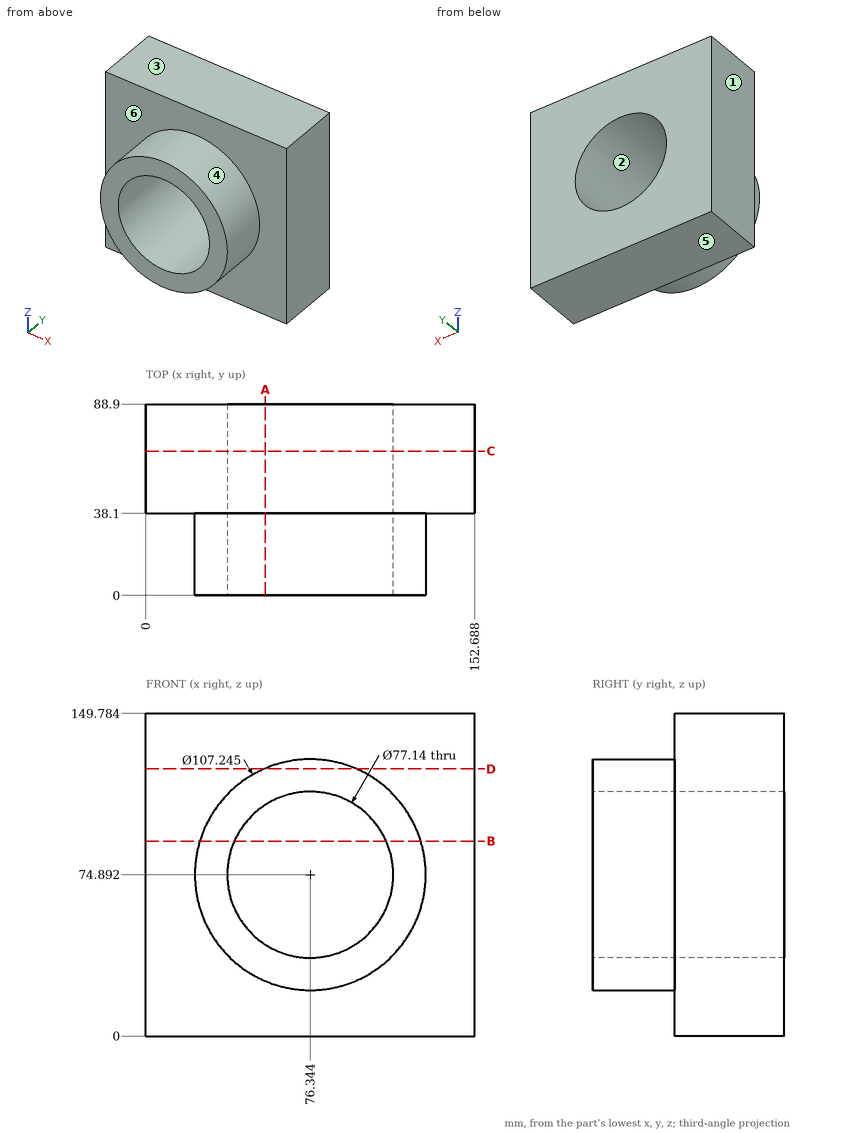
Can you work these out from the drawing? Everything is in mm from the part's minimum corner. A direction names the side the tool comes from. Coordinates: 2 decimals unless noted, no trailing zeros. Write each loop counter-clockwise with the first axis right and the second up, starting at its lowest first coordinate (ties: lowest second). Pieces come first, ordered by that corner, then holes. Notation, with made-up numbers: (39, 48) -> (55, 48) arc R15 cw to (55, 71) -> close; hole circle Ø10 at (82.25, 48.25). An arc over 180 degrees is marked (long way). Write each question's results on one line, items separated by ' | '. Start each with the question number.
Q1. Imagine slicing it at B-B (z = 90.5). Write out the boundary of the cut face in (x, y) (1 decimal).
Q2. If I drill on probe 1 along Z at (x, y) = (75.5, 28); probe 2 along Y at (x, z) = (75.5, 20); probe 3 along X at (y, z) = (56.5, 61) (1 decimal), over which ranges is the centre line in solid material (lowest first)?
Q3. Imagine slicing it at C-C (y = 67). Write out the boundary of the cut face in (x, z) (1 decimal), then the cut area to 3 significant figures.
Q4. Imagine slicing it at D-D (z = 124). Write out the boundary of the cut face in (x, y).
Q5. Imagine slicing it at A-A (x = 55.5). Write out the boundary of the cut face in (y, z) (1 decimal).
Q6. I'm going to push flat-ended pins straight in: pin 1 (8 mm diameter, centred on y = 13, z = 126.5, fed in from +X); pin 2 (5 mm diameter, centred on y = 12, z = 75, fed in from +X). Where does each tip first touch, or does it pass through?
Q7. On a 3-axis mill with a long thin cutter (end or side, diameter ignored), from which of +Z, -Z, +X, -X, +Y, -Y can I reach the whole of each face in a straight line? I mean the marked faces 5 and 6. Say none if no direction works.
Q8. We'd pull the mould along X, two halves only. Please class the marked faces 1, 2, 3 and 4: +X half, -X half, draft (parallel to the pull), parting line (faces both ways), or undercut.
Taken from the geometry:
1) outline: (0, 38.1) -> (25, 38.1) -> (25, 0) -> (41.1, 0) -> (41.1, 88.9) -> (0, 88.9) -> close; (111.6, 0) -> (127.6, 0) -> (127.6, 38.1) -> (152.7, 38.1) -> (152.7, 88.9) -> (111.6, 88.9) -> close
2) probe 1: z = 21.28 to 36.33, 113.45 to 128.51 | probe 2: y = 38.1 to 88.9 | probe 3: x = 0 to 40.4, 112.3 to 152.7
3) outline: (0, 0) -> (152.7, 0) -> (152.7, 149.8) -> (0, 149.8) -> close; hole circle Ø77.1 at (76.3, 74.9) | area: 18,200 mm^2
4) outline: (0, 38.1) -> (54.81, 38.1) -> (54.81, 0) -> (97.88, 0) -> (97.88, 38.1) -> (152.69, 38.1) -> (152.69, 88.9) -> (0, 88.9) -> close
5) outline: (0, 25.5) -> (38.1, 25.5) -> (38.1, 0) -> (88.9, 0) -> (88.9, 42.4) -> (0, 42.4) -> close; (0, 107.3) -> (88.9, 107.3) -> (88.9, 149.8) -> (38.1, 149.8) -> (38.1, 124.3) -> (0, 124.3) -> close
6) pin 1: stops at x = 101.02 | pin 2: stops at x = 129.97
7) face 5: -Z, +X, -X, +Y, -Y | face 6: -Y
8) face 1: -X half | face 2: undercut | face 3: draft | face 4: parting line
